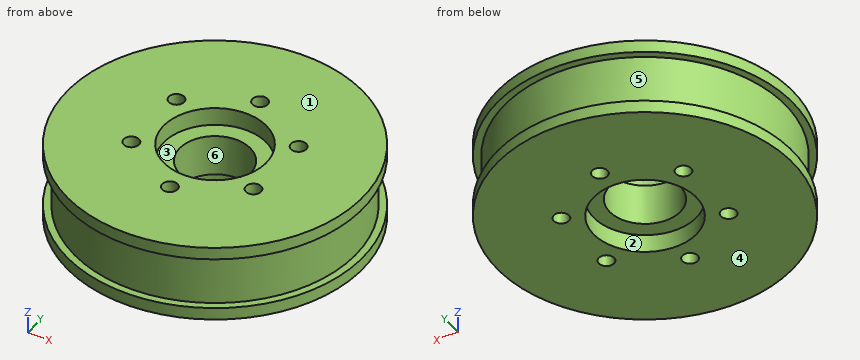
from build123d import *

# Parameters (mm, degrees)
SKETCH1_R             = 36.5125
BOSS_EXTRUDE1_DEPTH   = 19.05
SKETCH2_R             = 8.73125
CUT_EXTRUDE1_DEPTH    = 20.05
SKETCH3_R             = 12.7
CUT_EXTRUDE2_DEPTH    = 4.445
SKETCH4_R             = 12.7
CUT_EXTRUDE3_DEPTH    = 4.445
F_6_CLEARANCE_HOLE1_D = 3.7973


with BuildPart() as part:
    # Sketch1 → Boss-Extrude1 (new body)
    with BuildSketch(Plane.XY):
        Circle(SKETCH1_R)
    extrude(amount=BOSS_EXTRUDE1_DEPTH)

    # Sketch2 → Cut-Extrude1 (cut, through all)
    with BuildSketch(Plane.XY.offset(19.05)):
        Circle(SKETCH2_R)
    extrude(amount=-CUT_EXTRUDE1_DEPTH, mode=Mode.SUBTRACT)

    # Sketch3 → Cut-Extrude2 (cut)
    with BuildSketch(Plane.XY.offset(19.05)):
        Circle(SKETCH3_R)
    extrude(amount=-CUT_EXTRUDE2_DEPTH, mode=Mode.SUBTRACT)

    # Sketch4 → Cut-Extrude3 (cut)
    with BuildSketch(Plane(origin=(0, 0, 0), x_dir=(-1, 0, 0), z_dir=(0, 0, -1))):
        Circle(SKETCH4_R)
    extrude(amount=-CUT_EXTRUDE3_DEPTH, mode=Mode.SUBTRACT)

    # #6 Clearance Hole1 (through all)
    with Locations(Plane(origin=(-8.170302988, -47.003517203, 19.05), x_dir=(1, 0, 0), z_dir=(0, 0, 1))):
        with Locations((8.170302988, 64.758117203), (-7.205631646, 55.880817203), (-7.205631646, 38.126217203), (8.170302988, 29.248917203), (23.546237622, 38.126217203), (23.546237622, 55.880817203)):
            Hole(F_6_CLEARANCE_HOLE1_D / 2)

    # Sketch10 → Cut-Revolve1 (revolve, cut)
    with BuildSketch(Plane(origin=(0, 0, 0), x_dir=(0, 0, -1), z_dir=(1, 0, 0))):
        Polygon((-16.002, 36.5125), (-16.002, 34.7345), (-3.048, 34.7345), (-3.048, 36.5125), (-3.048, 51.152208686), (-16.002, 51.152208686), align=None)
    revolve(axis=Axis((0, 0, 19.05), (0, 0, -1)), mode=Mode.SUBTRACT)


solid = part.part
Verification items for the finished model (mm, model axes). Face numbers are marked on the shaded views. A direction names the side the tool comes from. Round coordinates to 2 decimals unless told otherwise and drop trailing zeros. Loops run counter-clockwise (first coordinate to the right, second up) from the corner with the lowest first, then second, coordinate; pieces in that order, holes last. Notation, with made-up numbers: (-13.5, 60) - (12.5, 60) arc R25 cw to (12.5, 94) - close; hole circle Ø5 at (83, 48). An arc over 180 degrees is marked (long way). Answer in a Markdown table with one row per item. Add a question column.
Q1. Tool access check on the marked faces 1, 2 and 3. Record the directions out of +Z, -Z, +X, -X, +Y, -Y that give a thin tool (end or side, any length) a straight path to the whole face; none if there is none.
Q2. Gauge pin test, flat ends, axial feed: pin 1 (4 mm diameter, centred on y = 26.5, z = 11, fed in from +X); pin 2 (20.5 mm diameter, centred on x = 0, y = 0, fed in from +Z) (3 decimals); pin 3 (2 mm diameter, centred on x = 22, z = 3, fed in from +Y). Record the tip position at first contact, or that the pin passes through.
Q3. Release check for a two-part mould opening along Y. For the marked faces 4, 5 and 6 record: pulls with the +Y half, pulls with the -Y half, needs draft (parallel to the pull), parting line crosses it, or undercut.
Q4. Section check C-C on z = 13.75. Enter the section's corners in (x, y).
Q5. Section check D-D on y = 30. Enter the section's corners in (x, z).
Q6. Section check B-B on x = 0. State how many separate pieces and enclosed holes the cut face has, plus the area to 3 significant figures.
Q7. Material ranges on line 1 (Z direction, x = -32.5, y = -12.5); line 2 (Y direction, x = -1, z = 12.25); line 3 (Y direction, x = -1.5, z = 3.5), recorded low to high.
Found:
| question | item | result |
|---|---|---|
| 1 | face 1 | +Z, +X, -X, +Y, -Y |
| 1 | face 2 | -Z |
| 1 | face 3 | +Z |
| 2 | pin 1 | stops at x = 24.62 |
| 2 | pin 2 | stops at z = 14.605 |
| 2 | pin 3 | stops at y = 29.87 |
| 3 | face 4 | needs draft |
| 3 | face 5 | parting line crosses it |
| 3 | face 6 | undercut |
| 4 | outline | circle Ø69.47 at (0, 0); hole circle Ø3.8 at (-15.38, -8.88); hole circle Ø3.8 at (-15.38, 8.88); hole circle Ø17.46 at (0, 0); hole circle Ø3.8 at (0, -17.75); hole circle Ø3.8 at (0, 17.75); hole circle Ø3.8 at (15.38, -8.88); hole circle Ø3.8 at (15.38, 8.88) |
| 5 | outline | (-20.81, 0) - (20.81, 0) - (20.81, 3.05) - (17.51, 3.05) - (17.51, 16) - (20.81, 16) - (20.81, 19.05) - (-20.81, 19.05) - (-20.81, 16) - (-17.51, 16) - (-17.51, 3.05) - (-20.81, 3.05) - close |
| 6 | separate pieces | 4 |
| 6 | enclosed holes | 0 |
| 6 | area | 797 mm² |
| 7 | line 1 | z = 0 to 3.05, 16 to 19.05 |
| 7 | line 2 | y = -34.72 to -19.37, -16.14 to -8.67, 8.67 to 16.14, 19.37 to 34.72 |
| 7 | line 3 | y = -34.7 to -18.92, -16.59 to -12.61, 12.61 to 16.59, 18.92 to 34.7 |
